Autodesk Inventor part; units mm, degrees
ref_plane "YZ Plane" through (0, 0, 0) normal (1, 0, 0) x (0, 1, 0)
ref_plane "XZ Plane" through (0, 0, 0) normal (0, 1, 0) x (-1, 0, 0)
ref_plane "XY Plane" through (0, 0, 0) normal (0, 0, 1) x (1, 0, 0)
sketch "Sketch1" plane through (0, 0, 0) normal (0, 1, 0) x (-1, 0, 0)
  line L0 (0, 0) -> (0, -452.12) construction
  circle A0 centre (0, -452.12) radius 6.35
  circle A1 centre (0, 0) radius 7.62
  circle A2 centre (0, 0) radius 29.337 construction
  circle A3 centre (0, 0) radius 35.687 construction
  circle A4 centre (0, -452.12) radius 19.05 construction
  circle A5 centre (0, 0) radius 23.8125 construction
  circle A6 centre (0, -23.8125) radius 2.413
  circle A7 centre (20.6222, -11.9063) radius 2.413
  circle A8 centre (20.6222, 11.9062) radius 2.413
  circle A9 centre (0, 23.8125) radius 2.413
  circle A10 centre (-20.6222, 11.9063) radius 2.413
  circle A11 centre (-20.6222, -11.9062) radius 2.413
  line L1 (35.6628, -1.3132) -> (19.0371, -452.821)
  line L2 (-35.6628, -1.3132) -> (-19.0371, -452.821)
  arc A12 (35.6628, -1.3132) -> (-35.6628, -1.3132) centre (0, 0) ccw
  arc A13 (-19.0371, -452.821) -> (19.0371, -452.821) centre (0, -452.12) ccw
  dimension "d6" = 47.625
  dimension "d0" = 452.12
  dimension "d1" = 12.7
  dimension "d2" = 15.24
  dimension "d3" = 58.674
  dimension "d4" = 6.35
  dimension "d5" = 12.7
  dimension "d7" = 4.826
  dimension "d10" = 360
extrude "Extrusion1" add sketch "Sketch1" along normal blind 6.35
properties part number "DragBarLinkage3 Bar1"
Work out the finished part from the listing and answer in its coordinate system (mm). Coordinates: 2 decimals unless noted, no trailing zeros. Loops run counter-clockwise (first coordinate to the right, second up) from the corner with the lowest first, then second, coordinate; pieces in that order, holes last. Notation, with made-up numbers: M -29,33.5 L 6,33.5 A31 cw 6,70.5 Z; hole C 36,-20 d10. An arc over 180 degrees is marked long. Answer in a Markdown table with one row per item. Add a question column.
1. Consider L1, parallel to Z at x = 0, y = 4; L2, parallel to X at y = 3.5, z = -452.12; L3, parallel to Z at x = -4.5, y = 5.75. Determine where each line is inside the solid, lowest interval first.
2. Find section B-B, the plane z = -50.5. Write down the section's boundary in (x, y).
3. The mould has two halves that part along Z. Classify faces 1 (the flat face through (0, 0, -158)), 2 (the cylindrical face through (-0.409, 3.131, -471.166)), 3 (the cylindrical face through (1.38, 3.13, -445.92)): pulls with the +Z half, pulls with the -Z half, needs draft (parallel to the pull), parting line crosses it, or undercut.
4. Find section A-A, the plane y = 1.5. State how many separate pieces and enclosed holes the cut face has, then the cut area to 3 significant figures.
5. Find section C-C, the plane z = -215. Write down the section's boundary in (x, y).
6. Flat-ended cylindrical pins translate along their axes: P1, Ø2, axis at y = 4, z = -124.5, coming from the -X side; P2, Ø3, axis at x = -27.5, y = 1, coming from the +Z side; P3, Ø4, axis at x = 20.62, z = 11.91, coming from the -Y side; P4, Ø1, axis at x = -12.5, y = 2, coming from the -Z side. Find the tip coordinate at first contact, or state that the pin passes through.
Reported:
| question | item | result |
|---|---|---|
| 1 | L1 | z = -471.17 to -458.47, -445.77 to -26.23, -21.4 to -7.62, 7.62 to 21.4, 26.23 to 35.69 |
| 1 | L2 | x = -19.06 to -6.35, 6.35 to 19.06 |
| 1 | L3 | z = -470.63 to -456.6, -447.64 to -6.15, 6.15 to 35.4 |
| 2 | outline | M -33.85,0 L 33.85,0 L 33.85,6.35 L -33.85,6.35 Z |
| 3 | face 1 | needs draft |
| 3 | face 2 | pulls with the -Z half |
| 3 | face 3 | undercut |
| 4 | separate pieces | 1 |
| 4 | enclosed holes | 8 |
| 4 | area | 26,900 mm^2 |
| 5 | outline | M -27.79,0 L 27.79,0 L 27.79,6.35 L -27.79,6.35 Z |
| 6 | P1 | stops at x = -31.16 |
| 6 | P2 | stops at z = 24.45 |
| 6 | P3 | passes through |
| 6 | P4 | stops at z = -466.92 |
